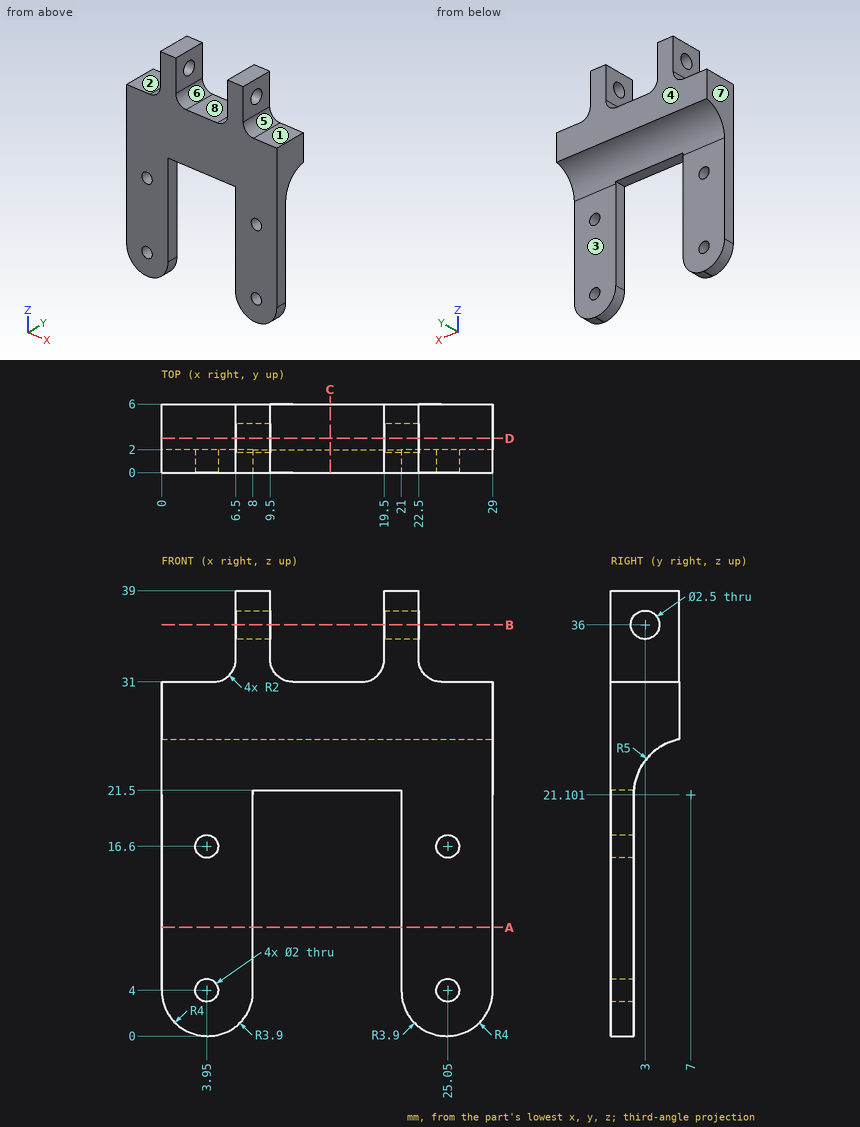
Drawing for the job (mm, zero at the part's lowest x, y, z). A direction names the side the tool comes from. Give positions to 0.01 mm unless a question says otherwise; leave off trailing zeros. Write each loop counter-clockwise with the first axis right and the second up, starting at its lowest first coordinate (ties: lowest second). Pieces come first, ordered by that corner, then holes. Notation, with made-up numbers: M 63,75.25 L 75,75.25 A14 ccw 75,81.25 Z; hole C -12.5,3 d11. An arc over 180 degrees is marked long. Use CSV: the item, a comma, the result in double quotes.
Item 1: Which spindle directions (+Z, -Z, +X, -X, +Y, -Y) get a long thin tool onto all of the face, cutting with end or side? Do the marked faces 1, 2, 3 and 4. Say none if no direction does.
Taken from the geometry:
face 1,"+Z, +X, +Y, -Y"
face 2,"+Z, -X, +Y, -Y"
face 3,"-Z, +X, -X, +Y"
face 4,"+Z, -Z, +X, -X, +Y"
Item 2: Slice it at D-D on y = 3. Write the cut outline in (x, z).
Taken from the geometry:
outline,"M 0,24.1 L 29,24.1 L 29,31 L 24.5,31 A2 cw 22.5,33 L 22.5,34.75 L 19.5,34.75 L 19.5,33 A2 cw 17.5,31 L 11.5,31 A2 cw 9.5,33 L 9.5,34.75 L 6.5,34.75 L 6.5,33 A2 cw 4.5,31 L 0,31 Z; M 6.5,37.25 L 9.5,37.25 L 9.5,39 L 6.5,39 Z; M 19.5,37.25 L 22.5,37.25 L 22.5,39 L 19.5,39 Z"
Item 3: Slice it at A-A on z = 9.5. Write the cut outline in (x, y), plus the area to 3 significant figures.
Taken from the geometry:
outline,"M 0,0 L 8,0 L 8,2 L 0,2 Z; M 21,0 L 29,0 L 29,2 L 21,2 Z"
area,"32.0 mm²"
Item 4: Drill centre lines: probe 1 along X at (y, z) = (1.25, 4); probe 2 along Y at (x, z) = (8.1, 36); probe 3 along X at (y, z) = (1, 33.5). Where is each one in solid material? Low to high.
Taken from the geometry:
probe 1,"x = 0 to 2.95, 4.95 to 8, 21 to 24.05, 26.05 to 29"
probe 2,"y = 0 to 1.75, 4.25 to 6"
probe 3,"x = 6.5 to 9.5, 19.5 to 22.5"
Item 5: Pin check, flat tips, straight feed: P1, Ø3, axis at x = 15, y = 1.5, coming from the +Z side; P2, Ø2.5, axis at x = 3.95, z = 16.6, coming from the -Y side; P3, Ø6.5, axis at x = 6, z = 11.5, coming from the +Y side; P4, Ø3, axis at y = 3, z = 36, coming from the +X side. Stop position of each tip, or through.
Taken from the geometry:
P1,"stops at z = 31"
P2,"stops at y = 0"
P3,"stops at y = 2"
P4,"stops at x = 22.5"
Item 6: Slice it at B-B on z = 36. Write the cut outline in (x, y).
Taken from the geometry:
outline,"M 6.5,0 L 9.5,0 L 9.5,1.75 L 6.5,1.75 Z; M 6.5,4.25 L 9.5,4.25 L 9.5,6 L 6.5,6 Z; M 19.5,0 L 22.5,0 L 22.5,1.75 L 19.5,1.75 Z; M 19.5,4.25 L 22.5,4.25 L 22.5,6 L 19.5,6 Z"
Item 7: Pull direction X, two halves, no side cores. Call the marked faces 5, 6, 7 and 8: +X half, -X half, draft (parallel to the pull), parting line (faces both ways), or undercut.
Taken from the geometry:
face 5,"+X half"
face 6,"undercut"
face 7,"-X half"
face 8,"undercut"
Item 8: Slice it at C-C on x = 14.75. Write the cut outline in (y, z), plus the area to 3 significant figures.
Taken from the geometry:
outline,"M 0,21.5 L 2.02,21.5 A5 cw 6,26 L 6,31 L 0,31 Z"
area,"43.9 mm²"
